from build123d import *

# Parameters (mm, degrees)
BOSS_EXTRUDE1_DEPTH      = 2
BOSS_EXTRUDE1_DEPTH_BACK = 1
SKETCH1_R                = 40
BOSS_EXTRUDE2_DEPTH      = 12
CIRPATTERN1_COUNT        = 5
SKETCH4_R                = 5
BOSS_EXTRUDE3_DEPTH      = 2


# Read off the part's stored shape, not the designer's step: Boss-Extrude2
with BuildPart() as part:
    # Sketch1 → Boss-Extrude1 (new, two sides: drawn at the far end of the back side and taken through both)
    with BuildSketch(Plane(origin=(0, 0, 0), x_dir=(1, 0, 0), z_dir=(0, 1, 0)).offset(-BOSS_EXTRUDE1_DEPTH_BACK)):
        with Locations(Location((0, 0, 0), (0, 0, 270))):
            Circle(SKETCH1_R)
    extrude(amount=BOSS_EXTRUDE1_DEPTH + BOSS_EXTRUDE1_DEPTH_BACK)

    # Boss-Extrude2 outline → Boss-Extrude2 (add)
    with BuildSketch(Plane(origin=(0, 2, 0), x_dir=(1, 0, 0), z_dir=(0, 1, 0))):
        with BuildLine():
            add(Edge.make_bspline(
                [(-1.648457537, 7.469358199), (-2.104873805, 7.937868262), (-3.086385024, 8.83695283), (-5.118879824, 10.300544164), (-7.85339222, 11.617216343), (-11.343679645, 12.411124094), (-16.177419051, 12.495643266), (-22.32154029, 10.877489917), (-29.038746805, 6.570733882), (-33.401405456, 1.389922557), (-35.761319101, -3.474155864), (-36.874262221, -7.426752725), (-37.238472583, -11.634394908), (-36.915436622, -14.613747914), (-36.587236294, -16.149943806), (-36.580010635, -16.183411937)],
                knots=[0, 0, 0, 0, 0.03125, 0.0625, 0.125, 0.1875, 0.25, 0.375, 0.5, 0.625, 0.6875, 0.75, 0.8125, 0.875, 0.876391371, 0.876391371, 0.876391371, 0.876391371], degree=3))
            Line((-1.648457537, 7.469358199), (-0.215875004, 8.864961038))
            add(Edge.make_bspline(
                [(-0.215875004, 8.864961038), (-0.725572372, 9.388164005), (-1.819134041, 10.389961885), (-4.104895535, 12.036976258), (-7.191277155, 13.522686378), (-11.109594838, 14.411975027), (-16.471086792, 14.501770787), (-23.156943321, 12.729175608), (-30.376376148, 8.096753493), (-35.077876345, 2.519665418), (-37.639776615, -2.757260327), (-38.616179028, -6.222859697), (-38.916318413, -8.348122546), (-38.979627679, -8.9771168)],
                knots=[0, 0, 0, 0, 0.03125, 0.0625, 0.125, 0.1875, 0.25, 0.375, 0.5, 0.625, 0.6875, 0.75, 0.775839178, 0.775839178, 0.775839178, 0.775839178], degree=3))
            ThreePointArc((-38.979627679, -8.9771168), (-37.951250413, -12.637349092), (-36.580010635, -16.183411937))
        make_face()
    boss_extrude2 = extrude(amount=BOSS_EXTRUDE2_DEPTH)

    # CirPattern1: Boss-Extrude2 ×5 about axis
    cirpattern1_axis = Axis((0, 0, 0), (0, -1, 0))
    for i in range(1, CIRPATTERN1_COUNT):
        add(boss_extrude2.rotate(cirpattern1_axis, i * 360 / CIRPATTERN1_COUNT))

    # Sketch3 → Cut-Revolve1 (revolve, cut)
    with BuildSketch(Plane.XY, mode=Mode.PRIVATE) as cut_revolve1_sk:
        Polygon((0, 2), (-9, 2), (-13.731613045, 15), (0, 15), align=None)
    revolve(cut_revolve1_sk.sketch.rotate(Axis((0, 15, 0), (0, -1, 0)), 270), axis=Axis((0, 15, 0), (0, -1, 0)), mode=Mode.SUBTRACT)

    # Sketch4 → Boss-Extrude3 (add)
    with BuildSketch(Plane(origin=(0, 2, 0), x_dir=(1, 0, 0), z_dir=(0, 1, 0))):
        with Locations(Location((0, 0, 0), (0, 0, 270))):
            Circle(SKETCH4_R)
    extrude(amount=BOSS_EXTRUDE3_DEPTH)


solid = part.part
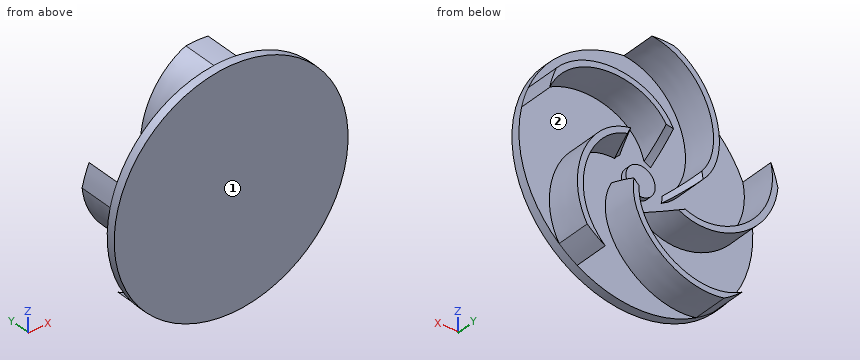
Read the model definition and answer for the solid it produces. Units are mm, in the model's axes. Face numbers are marked on the shaded views. Round coordinates to 2 decimals unless told otherwise and drop trailing zeros.
1) Flat-ended cylindrical pins translate along their axes: pin 1 (3 mm diameter, centred on x = -5, z = 11, fed in from +Y); pin 2 (5 mm diameter, centred on y = 0.5, z = -23.5, fed in from -X); pin 3 (8 mm diameter, centred on x = -24.5, y = 12.5, fed in from +Z); pin 4 (6 mm diameter, centred on x = 18, z = 19.5, fed in from +Y). Find the tip coordinate at first contact, or state that the pin passes through.
2) The part is cut by section A-A on y = 3. Give the number of separate pieces and of enclosed holes in the cut face, plus the area to 3 significant figures.
3) Straight lines are drawn through the part: L1, parallel to X at y = 8.25, z = -6.5; L2, parallel to Z at x = 0, y = 5.25; L3, parallel to X at y = 10.75, z = -8. For each, find the intervals that lie inside material, in ascending order.
4) The mould has two halves that part along X. Classify the marked faces 1 and 2: released by +X, released by -X, zero draft, split by the parting line, or undercut.
Resolved:
1. pin 1: stops at y = 11.48
1. pin 2: stops at x = -34.04
1. pin 3: stops at z = -6.51
1. pin 4: stops at y = 14
2. separate pieces: 6
2. enclosed holes: 0
2. area: 599 mm2
3. L1: x = -31.45 to -28.51, 9.21 to 9.8, 25.14 to 27.33
3. L2: z = -29.78 to -27.28, 14.44 to 17.5, 39 to 40
3. L3: x = -29.83 to -26.58, 9.19 to 10.16, 25.78 to 27.92
4. face 1: zero draft
4. face 2: undercut
